```python
from build123d import *

# Parameters (mm, degrees)
SKETCH1_W           = 68.5
SKETCH1_H           = 53.5
SKETCH1_R           = 1.75
BOSS_EXTRUDE1_DEPTH = 0.8
SKETCH2_W           = 20
SKETCH2_H           = 8
BOSS_EXTRUDE2_DEPTH = 20
SKETCH3_W           = 16
SKETCH3_H           = 3
CUT_EXTRUDE1_DEPTH  = 7


with BuildPart() as part:
    # Sketch1 → Boss-Extrude1 (new body, symmetric)
    with BuildSketch(Plane.XY):
        Rectangle(SKETCH1_W, SKETCH1_H)
        with Locations((-30, 22.5)):
            Circle(SKETCH1_R, mode=Mode.SUBTRACT)
        with Locations((30, 22.5)):
            Circle(SKETCH1_R, mode=Mode.SUBTRACT)
        with Locations((-30, -22.5)):
            Circle(SKETCH1_R, mode=Mode.SUBTRACT)
        with Locations((30, -22.5)):
            Circle(SKETCH1_R, mode=Mode.SUBTRACT)
    extrude(amount=BOSS_EXTRUDE1_DEPTH, both=True)

    # Sketch2 → Boss-Extrude2 (add)
    with BuildSketch(Plane.XY.offset(0.8)):
        with Locations((-12.399398806, -18.931036611)):
            Rectangle(SKETCH2_W, SKETCH2_H)
        with Locations((12.039766375, -18.931036611)):
            Rectangle(SKETCH2_W, SKETCH2_H)
    extrude(amount=BOSS_EXTRUDE2_DEPTH)

    # Sketch3 → Cut-Extrude1 (cut)
    with BuildSketch(Plane.XY.offset(20.8)):
        with Locations((-12.399398806, -16.431036611)):
            Rectangle(SKETCH3_W, SKETCH3_H)
        with Locations((-12.399398806, -21.431036611)):
            Rectangle(SKETCH3_W, SKETCH3_H)
        with Locations((12.039766375, -16.431036611)):
            Rectangle(SKETCH3_W, SKETCH3_H)
        with Locations((12.039766375, -21.431036611)):
            Rectangle(SKETCH3_W, SKETCH3_H)
    extrude(amount=-CUT_EXTRUDE1_DEPTH, mode=Mode.SUBTRACT)


solid = part.part
```
Model file for the job. Use its own axes, mm. A direction names the side the tool comes from. Give positions to 0.01 mm unless a question says otherwise; leave off trailing zeros. Loops run counter-clockwise (first coordinate to the right, second up) from the corner with the lowest first, then second, coordinate; pieces in that order, holes last. Notation, with made-up numbers: (20, -24.5) - (39, -24.5) arc R19 cw to (39, 5.5) - close; hole circle Ø7 at (-30.75, 78.25). An arc over 180 degrees is marked (long way). One line per item, written item: value. Start each with the question number.
1. Slice it at B-B (y = 22.5). List the corners of the cut face in (x, z), plus the area to 3 significant figures.
2. Slice it at A-A (z = 10.5). List the corners of the cut face in (x, y), plus the area to 3 significant figures.
3. Slice it at D-D (z = 15). List the corners of the cut face in (x, y), plus the area to 3 significant figures.
4. Pin check, flat tips, straight feed: pin 1 (5 mm diameter, centred on x = 25.5, z = 4.5, fed in from -Y); pin 2 (1.5 mm diameter, centred on x = 3, z = 6.5, fed in from -Y); pin 3 (2.5 mm diameter, centred on y = -21, z = 16, fed in from -X); pin 4 (3.5 mm diameter, centred on x = -9.5, z = 18, fed in from +Y). Stop position of each tip, or through.
5. Which spindle directions (+Z, -Z, +X, -X, +Y, -Y) get a long thin tool onto all of the face, cutting with end or side? Do faces 5 (the flat face through (-13, -14.931, 8)), 6 (the flat face through (4.04, -16, 17)), 7 (the flat face through (-2.399, -19, 11)), 8 (the flat face through (20.04, -21, 17)). Say none if no direction does.
6. Probe L1, parallel to Y at x = 30, z = 0.15; L2, parallel to Z at x = 29, y = -11.5; L3, parallel to Y at x = 11, z = 13. List the from-to ranges inside material, lowest first. Write a range as from..to.
7. Slice it at C-C (x = -8.5). List the corners of the cut face in (y, z).
8. Pull direction Y, two halves, no side cores. Call faces 1 (the flat face through (12, -19.931, 17)), 2 (the cylindrical face through (28.71, 23.68, -0.01)), 3 (the flat face through (-13, -21, 13.8)), 4 (the flat face through (-13, -17.931, 17)): pulls with the +Y half, pulls with the -Y half, needs draft (parallel to the pull), parting line crosses it, or undercut.
Solution:
1. outline: (-34.25, -0.8) - (-31.75, -0.8) - (-31.75, 0.8) - (-34.25, 0.8) - close; (-28.25, -0.8) - (28.25, -0.8) - (28.25, 0.8) - (-28.25, 0.8) - close; (31.75, -0.8) - (34.25, -0.8) - (34.25, 0.8) - (31.75, 0.8) - close
1. area: 98.4 mm^2
2. outline: (-22.4, -22.93) - (-2.4, -22.93) - (-2.4, -14.93) - (-22.4, -14.93) - close; (2.04, -22.93) - (22.04, -22.93) - (22.04, -14.93) - (2.04, -14.93) - close
2. area: 320 mm^2
3. outline: (-22.4, -22.93) - (-20.4, -22.93) - (-20.4, -19.93) - (-4.4, -19.93) - (-4.4, -22.93) - (-2.4, -22.93) - (-2.4, -14.93) - (-4.4, -14.93) - (-4.4, -17.93) - (-20.4, -17.93) - (-20.4, -14.93) - (-22.4, -14.93) - close; (2.04, -22.93) - (4.04, -22.93) - (4.04, -19.93) - (20.04, -19.93) - (20.04, -22.93) - (22.04, -22.93) - (22.04, -14.93) - (20.04, -14.93) - (20.04, -17.93) - (4.04, -17.93) - (4.04, -14.93) - (2.04, -14.93) - close
3. area: 128 mm^2
4. pin 1: passes through
4. pin 2: stops at y = -22.93
4. pin 3: stops at x = -22.4
4. pin 4: stops at y = -17.93
5. face 5: +Z, +X, -X, +Y
5. face 6: +Z, +Y
5. face 7: +Z, +Y, -Y
5. face 8: +Z, -Y
6. L1: y = -26.75..-24.25, -20.75..20.75, 24.25..26.75
6. L2: z = -0.8..0.8
6. L3: y = -22.93..-14.93
7. outline: (-26.75, -0.8) - (26.75, -0.8) - (26.75, 0.8) - (-14.93, 0.8) - (-14.93, 13.8) - (-17.93, 13.8) - (-17.93, 20.8) - (-19.93, 20.8) - (-19.93, 13.8) - (-22.93, 13.8) - (-22.93, 0.8) - (-26.75, 0.8) - close
8. face 1: pulls with the -Y half
8. face 2: undercut
8. face 3: needs draft
8. face 4: pulls with the +Y half
